The model under review builds one solid part; all positions refer to its coordinate system, in mm. A direction names the side the tool comes from. Round coordinates to 2 decimals unless told otherwise and drop trailing zeros. Write each loop counter-clockwise with the first axis right and the second up, starting at its lowest first coordinate (ties: lowest second). Pieces come first, ordered by that corner, then holes. Notation, with made-up numbers: M 20,11 L 35,11 A12 cw 35,18 Z; hole C 64.25,64 d3. An arc over 180 degrees is marked long. One line per item, written item: value. Start each with the question number.
1) For P1, Ø4, axis at y = 17, z = 3.5, coming from the -X side; P2, Ø6, axis at x = -36, z = 20, coming from the +Y side; P3, Ø5, axis at x = -16.5, y = 18.5, coming from the +Z side; P4, Ø13, axis at x = -27.5, y = 36.5, coming from the -Z side, all flat-tipped, find the tip position at first contact; note any pin that passes through.
2) Tool access review of faces 1 (the face through (-16.964, 33, 4)), 2 (the face through (-15, 71, -2)), 3 (the face through (-15, 45, 8)), 4 (the face through (-13.964, 28, 6)), 5 (the face through (-24, -4.779, 18)): name each direction out of +Z, -Z, +X, -X, +Y, -Y from which nothing blocks a thin tool from reaching the whole face with its end or side.
3) Take a section at A-A, the plane x = -19. Write out the cut boundary in (y, z).
4) Take a section at C-C, the plane x = -25.5. Write out the cut boundary in (y, z), and give its area (3 significant figures).
5) Mouldability with a two-part tool opening along Y and no side actions: class faces 6 (the face through (-45.625, -3.258, 18.241)), 7 (the face through (-15.14, 73.7, -12.14)), 8 (the face through (-16, 23, 0)) as +Y half, -Y half, draft (parallel to the pull), parting line (faces both ways), or undercut.
6) Wall thickness on probe 1 along Z at (x, y) = (-14.5, 51.5); probe 2 along Y at (x, z) = (-23, 31); probe 3 along Y at (x, z) = (-14, -9.5): over which ranges is each line inside the solid? List them lowest first.
7) Take a section at B-B, the plane z = 18.5. Write out the cut boundary in (x, y), and give its area (3 significant figures).
from build123d import *
from build123d.topology import SkipClean

# Parameters (mm, degrees)
EXTRUDE_1_DEPTH     = 37
SKETCH_8_W          = 29
SKETCH_8_H          = 78
CUT_EXTRUDE_3_DEPTH = 10
EXTRUDE_START       = 22
SKETCH_10_R         = 5
EXTRUDE_4_DEPTH     = 22
SKETCH_11_R         = 2.5
CUT_EXTRUDE_4_DEPTH = 20


with BuildPart() as part:
    # 草图1 → 凸台-拉伸1 (new body)
    with BuildSketch(Plane.XY):
        with BuildLine():
            Line((-19.714285714, -1.778812154), (-56.964285714, -1.778812154))
            Line((-56.964285714, -1.778812154), (-33.964285714, -4.778812154))
            Line((-33.964285714, -4.778812154), (-13.964285714, -4.778812154))
            Line((-13.964285714, -4.778812154), (-13.964285714, 66.451491839))
            ThreePointArc((-13.964285714, 66.451491839), (-15.464285714, 76.221187846), (-16.964285714, 66.451491839))
            Line((-16.964285714, 66.451491839), (-16.964285714, -1.778812154))
            Line((-16.964285714, -1.778812154), (-19.714285714, -1.778812154))
        make_face()
    extrude(amount=EXTRUDE_1_DEPTH)

    # 草图8 → 切除-拉伸3 (cut, symmetric)
    with BuildSketch(Plane(origin=(-13.964285714, 0, 0), x_dir=(0, 0, -1), z_dir=(1, 0, 0))):
        with Locations((-22.5, 37.221187846)):
            Rectangle(SKETCH_8_W, SKETCH_8_H)
    extrude(amount=CUT_EXTRUDE_3_DEPTH, both=True, mode=Mode.SUBTRACT)

    # 草图10 → 凸台-拉伸4 (add)
    with SkipClean():  # the faces are left unmerged after this step: merging them gives an invalid solid
        with BuildSketch(Plane(origin=(0, 0, 0), x_dir=(-1, 0, 0), z_dir=(0, 0, -1)).offset(EXTRUDE_START)):
            with Locations((15.464285714, 71.221187846)):
                Circle(SKETCH_10_R)
        extrude(amount=-EXTRUDE_4_DEPTH)

    # 草图11 → 切除-拉伸4 (cut)
    with SkipClean():  # the faces are left unmerged after this step: merging them gives an invalid solid
        with BuildSketch(Plane(origin=(0, 0, -22), x_dir=(-1, 0, 0), z_dir=(0, 0, -1))):
            with Locations((15.464285714, 71.221187846)):
                Circle(SKETCH_11_R)
        extrude(amount=-CUT_EXTRUDE_4_DEPTH, mode=Mode.SUBTRACT)


solid = part.part
Checked values:
1. P1: stops at x = -16.96
1. P2: stops at y = -1.78
1. P3: stops at z = 8
1. P4: passes through
2. face 1: +Z, -Z, -X
2. face 2: -Z
2. face 3: +Z, +X, -X, +Y
2. face 4: +Z, -Z, +X, -Y
2. face 5: +Z, -Z, +X, -X, -Y
3. outline: M -4.78,0 L -1.78,0 L -1.78,37 L -4.78,37 Z; M 67.69,-22 L 74.76,-22 L 74.76,8 L 67.69,8 Z
4. outline: M -4.78,0 L -1.78,0 L -1.78,37 L -4.78,37 Z
4. area: 111 mm2
5. face 6: -Y half
5. face 7: undercut
5. face 8: draft
6. probe 1: z = 0 to 8
6. probe 2: y = -4.78 to -1.78
6. probe 3: y = 66.44 to 69.19, 73.25 to 76
7. outline: M -56.96,-1.78 L -33.96,-4.78 L -13.96,-4.78 L -13.96,-1.78 Z
7. area: 94.5 mm2
